```python
from build123d import *

# Parameters (mm, degrees)
SKETCH_1_R          = 12.5
SKETCH_1_R_2        = 10
EXTRUDE_1_DEPTH     = 30
SKETCH_2_W          = 3
SKETCH_2_H          = 32
EXTRUDE_2_DEPTH     = 30
CUT_EXTRUDE_2_DEPTH = 0.5
SKETCH_5_R          = 1.5
CUT_EXTRUDE_3_DEPTH = 42.617304093
FILLET_1_R          = 3


with BuildPart() as part:
    # 草图1 → 凸台-拉伸1 (new body)
    with BuildSketch(Plane(origin=(0, 0, 0), x_dir=(1, 0, 0), z_dir=(0, 1, 0))):
        with Locations(Location((0, 0, 0), (0, 0, 270))):
            Circle(SKETCH_1_R)
        with Locations(Location((0, 0, 0), (0, 0, 270))):
            Circle(SKETCH_1_R_2, mode=Mode.SUBTRACT)
    extrude(amount=EXTRUDE_1_DEPTH)

    # 草图2 → 凸台-拉伸2 (add)
    with BuildSketch(Plane(origin=(0, 0, 0), x_dir=(1, 0, 0), z_dir=(0, 1, 0))):
        with Locations((12.5, 0)):
            Rectangle(SKETCH_2_W, SKETCH_2_H)
    extrude(amount=EXTRUDE_2_DEPTH)

    # 草图4 → 切除-拉伸2 (cut)
    with BuildSketch(Plane.ZY.offset(-11)):
        Polygon((15.216666667, 27), (14.008333333, 29.092894726), (11.591666667, 29.092894726), (10.383333333, 27), (11.591666667, 24.907105274), (14.008333333, 24.907105274), align=None)
        Polygon((-10.78933236, 1.659293687), (-12.955751906, 0.588357588), (-14.966419546, 1.929063901), (-14.81066764, 4.340706313), (-12.644248094, 5.411642412), (-10.633580454, 4.070936099), align=None)
        Polygon((12.955751906, 0.588357588), (14.966419546, 1.929063901), (14.81066764, 4.340706313), (12.644248094, 5.411642412), (10.633580454, 4.070936099), (10.78933236, 1.659293687), align=None)
        Polygon((-14.008333333, 24.907105274), (-15.216666667, 27), (-14.008333333, 29.092894726), (-11.591666667, 29.092894726), (-10.383333333, 27), (-11.591666667, 24.907105274), align=None)
    extrude(amount=-CUT_EXTRUDE_2_DEPTH, mode=Mode.SUBTRACT)

    # 草图5 → 切除-拉伸3 (cut, through all)
    with BuildSketch(Plane.ZY.offset(-11.5)):
        with Locations(Location((-13, 27, 0), (0, 0, 270))):
            Circle(SKETCH_5_R)
        with Locations(Location((13, 27, 0), (0, 0, 270))):
            Circle(SKETCH_5_R)
        with Locations(Location((13, 3, 0), (0, 0, 270))):
            Circle(SKETCH_5_R)
        with Locations(Location((-13, 3, 0), (0, 0, 270))):
            Circle(SKETCH_5_R)
    extrude(amount=-CUT_EXTRUDE_3_DEPTH, mode=Mode.SUBTRACT)

    # 圆角1
    fillet_1_edges = [part.edges().sort_by_distance(p)[0] for p in [
        (12.5, 30, 16),
        (12.5, 30, -16),
        (12.5, 0, -16),
        (12.5, 0, 16),
    ]]
    fillet(fillet_1_edges, radius=FILLET_1_R)


solid = part.part
```
Input: part model. Units: mm. Frame: model coordinates. A direction names the side the tool comes from. Coordinates: 2 decimals unless noted, no trailing zeros. Loops run counter-clockwise (first coordinate to the right, second up) from the corner with the lowest first, then second, coordinate; pieces in that order, holes last. Notation, with made-up numbers: (26.5, -7) -> (68.5, -7) arc R25 ccw to (68.5, 27) -> close; hole circle Ø8 at (35, 73). An arc over 180 degrees is marked (long way). Use a Markdown table: item, result.
1) Cut plane D-D (z = -7). Return the cut outline in (x, y), then the cut area to 3 significant figures.
Results found:
| item | result |
|---|---|
| outline | (-10.36, 0) -> (-7.14, 0) -> (-7.14, 30) -> (-10.36, 30) -> close; (7.14, 0) -> (10.36, 0) -> (10.36, 30) -> (7.14, 30) -> close; (11, 0) -> (14, 0) -> (14, 30) -> (11, 30) -> close |
| area | 283 mm2 |
2) Cut plane A-A (z = 0). Return the cut outline in (x, y).
Results found:
| item | result |
|---|---|
| outline | (-12.5, 0) -> (-10, 0) -> (-10, 30) -> (-12.5, 30) -> close; (10, 0) -> (14, 0) -> (14, 30) -> (10, 30) -> close |
3) Contact query for flat-ended pins moving along their axis: pin 1 (2 mm diameter, centred on y = 3, z = 12, fed in from -X); pin 2 (4.5 mm diameter, centred on y = 26, z = 12, fed in from -X); pin 3 (4 mm diameter, centred on y = 24.5, z = -11, fed in from -X). Output: stop coordinate, or through.
Results found:
| item | result |
|---|---|
| pin 1 | stops at x = -5.94 |
| pin 2 | stops at x = -7.82 |
| pin 3 | stops at x = -8.67 |
4) Material intervals for line 1 along Z through (x, y) = (13.45, 27); line 2 along X through (y, z) = (6.25, 0); line 3 along X through (y, z) = (15, 7), sorted ascending. Write a range as from..to.
Results found:
| item | result |
|---|---|
| line 1 | z = -16..-14.5, -11.5..11.5, 14.5..16 |
| line 2 | x = -12.5..-10, 10..14 |
| line 3 | x = -10.36..-7.14, 7.14..10.36, 11..14 |
5) Access query for faces 1 (the cylindrical face through (12.73, 28.5, 13.07)), 2 (the flat face through (11.246, 25.939, -14.604)), 3 (the flat face through (11.246, 28.061, -10.996)). Directions: +Z, -Z, +X, -X, +Y, -Y. A direction counts if a zero-diameter tool reaches every point of the face in a straight line with its end or side. Return the directions, or none.
Results found:
| item | result |
|---|---|
| face 1 | +X |
| face 2 | -X |
| face 3 | none |
6) Cut plane C-C (y = 17). Return the cut outline in (x, z), then the cut area to 3 significant figures.
Results found:
| item | result |
|---|---|
| outline | (11, -16) -> (14, -16) -> (14, 16) -> (11, 16) -> (11, 5.94) arc R12.5 ccw (long way) to (11, -5.94) -> close; hole circle Ø20 at (0, 0) |
| area | 261 mm2 |
7) Cut plane B-B (x = 0). Return the cut outline in (y, z).
Results found:
| item | result |
|---|---|
| outline | (0, -12.5) -> (30, -12.5) -> (30, -10) -> (0, -10) -> close; (0, 10) -> (30, 10) -> (30, 12.5) -> (0, 12.5) -> close |
8) Pull-direction query (Y, two-part tool) for faces 4 (the cylindrical face through (12.52, 29.14, -15.1)), 5 (the flat face through (11.25, 4.87, -13.74)), 6 (the cylindrical face through (12.52, 0.86, 15.1)); classes: released by +Y, released by -Y, zero draft, split by the parting line, or undercut.
Results found:
| item | result |
|---|---|
| face 4 | released by +Y |
| face 5 | undercut |
| face 6 | released by -Y |
